Could you check a few things on this model? Use its own coordinates, in mm. Coordinates: 2 decimals unless noted, no trailing zeros. Loops run counter-clockwise (first coordinate to the right, second up) from the corner with the lowest first, then second, coordinate; pieces in that order, holes last. Notation, with made-up numbers: (0, 72.25) -> (24, 72.25) arc R14 cw to (24, 78.25) -> close; hole circle Ø4 at (57.5, -32). An arc over 180 degrees is marked (long way). One line per question, with ' | ' between items. Start each with the question number.
(1) Suppose I cut it at A-A (z = 186). Please give me the cut outline in (x, y).
(2) If I drill on line 1 along X through (y, z) = (0.75, 186); line 2 along Z through (x, y) = (-7, 1.75); line 3 along Z through (x, y) = (-2, 2.5), over which ranges is the centre line in solid material (lowest first)?
(3) I'm going to push flat-ended pins straight in: pin 1 Ø3 at (x, y) = (6.5, -5) entering from -Z; pin 2 Ø6 at (x, z) = (0.5, 187.5) entering from -Y. Where does each tip first touch, or does it pass through?
(4) Suppose I cut it at D-D (z = 63). Please give me the cut outline in (x, y), plus the area to 3 significant figures.
(5) Suppose I cut it at B-B (y = 0). Please give me the cut outline in (x, z).
(6) Suppose I cut it at C-C (x = 0). Please give me the cut outline in (y, z).
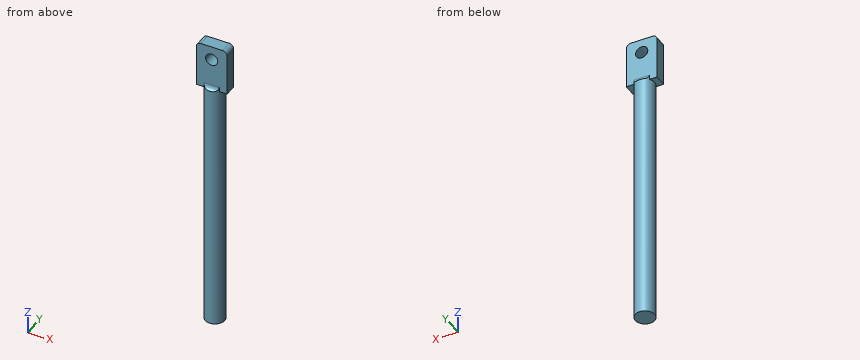
```python
from build123d import *

# Parameters (mm, degrees)
CROQUIS1_R              = 6.35
SALIENTE_EXTRUIR1_DEPTH = 165
CROQUIS2_W              = 20
CROQUIS2_H              = 8
SALIENTE_EXTRUIR2_DEPTH = 30
REDONDEO1_R             = 3
REDONDEO2_R             = 3
CROQUIS3_R              = 3.96875
CORTAR_EXTRUIR1_DEPTH   = 30
REDONDEO3_R             = 3


with BuildPart() as part:
    # Croquis1 → Saliente-Extruir1 (new body)
    with BuildSketch(Plane.XY):
        Circle(CROQUIS1_R)
    extrude(amount=SALIENTE_EXTRUIR1_DEPTH)

    # Croquis2 → Saliente-Extruir2 (add)
    with BuildSketch(Plane.XY.offset(165)):
        Rectangle(CROQUIS2_W, CROQUIS2_H)
    extrude(amount=SALIENTE_EXTRUIR2_DEPTH)

    # Redondeo1
    # the kernel refuses this fillet: 3 mm, written as the material it adds along each edge
    with BuildSketch(Plane(origin=(12.431784667, 4, 165), x_dir=(0, 1, 0), z_dir=(-1, 0, 0))) as redondeo1_piece_1_section:
        with BuildLine():
            CenterArc((REDONDEO1_R, -REDONDEO1_R), REDONDEO1_R, 90, 90)
            Line((0, -REDONDEO1_R), (0, 0))
            Line((0, 0), (REDONDEO1_R, 0))
        make_face()
    redondeo1_piece_1 = extrude(amount=24.863569334, mode=Mode.PRIVATE)
    redondeo1_piece_1 = redondeo1_piece_1 & Plane(origin=(0, 0, 165.727834691), x_dir=(1, 0, 0), z_dir=(0, 0, -1)) * Cylinder(6.35, 62, mode=Mode.PRIVATE)
    add(redondeo1_piece_1)

    # Redondeo2
    # the kernel refuses this fillet: 3 mm, written as the material it adds along each edge
    with BuildSketch(Plane(origin=(-12.431784667, -4, 165), x_dir=(0, 0, 1), z_dir=(1, 0, 0))) as redondeo2_piece_1_section:
        with BuildLine():
            CenterArc((REDONDEO2_R, REDONDEO2_R), REDONDEO2_R, 180, 90)
            Line((0, REDONDEO2_R), (0, 0))
            Line((0, 0), (REDONDEO2_R, 0))
        make_face()
    redondeo2_piece_1 = extrude(amount=24.863569334, mode=Mode.PRIVATE)
    redondeo2_piece_1 = redondeo2_piece_1 & Plane(origin=(0, 0, 165.727832958), x_dir=(1, 0, 0), z_dir=(0, 0, -1)) * Cylinder(6.35, 62, mode=Mode.PRIVATE)
    add(redondeo2_piece_1)

    # Croquis3 → Cortar-Extruir1 (cut)
    with BuildSketch(Plane.XZ.offset(4)):
        with Locations(Location((0, 186, 0), (0, 0, 270))):
            Circle(CROQUIS3_R)
    extrude(amount=-CORTAR_EXTRUIR1_DEPTH, mode=Mode.SUBTRACT)

    # Redondeo3
    redondeo3_edges = [part.edges().sort_by_distance(p)[0] for p in [
        (10, 0, 195),
        (-10, 0, 195),
    ]]
    fillet(redondeo3_edges, radius=REDONDEO3_R)


solid = part.part
```
Checks:
1) outline: (-10, -4) -> (-3.97, -4) -> (-3.97, 4) -> (-10, 4) -> close; (3.97, -4) -> (10, -4) -> (10, 4) -> (3.97, 4) -> close
2) line 1: x = -10 to -3.97, 3.97 to 10 | line 2: z = 165 to 195 | line 3: z = 0 to 182.57, 189.43 to 195
3) pin 1: stops at z = 165 | pin 2: stops at y = -4
4) outline: circle Ø12.7 at (0, 0) | area: 127 mm^2
5) outline: (-10, 165) -> (-6.35, 165) -> (-6.35, 0) -> (6.35, 0) -> (6.35, 165) -> (10, 165) -> (10, 192) arc R3 ccw to (7, 195) -> (-7, 195) arc R3 ccw to (-10, 192) -> close; hole circle Ø7.94 at (0, 186)
6) outline: (-6.35, 0) -> (6.35, 0) -> (6.35, 165.07) arc R3 cw to (4, 168) -> (4, 182.03) -> (-4, 182.03) -> (-4, 168) arc R3 cw to (-6.35, 165.07) -> close; (-4, 189.97) -> (4, 189.97) -> (4, 195) -> (-4, 195) -> close
